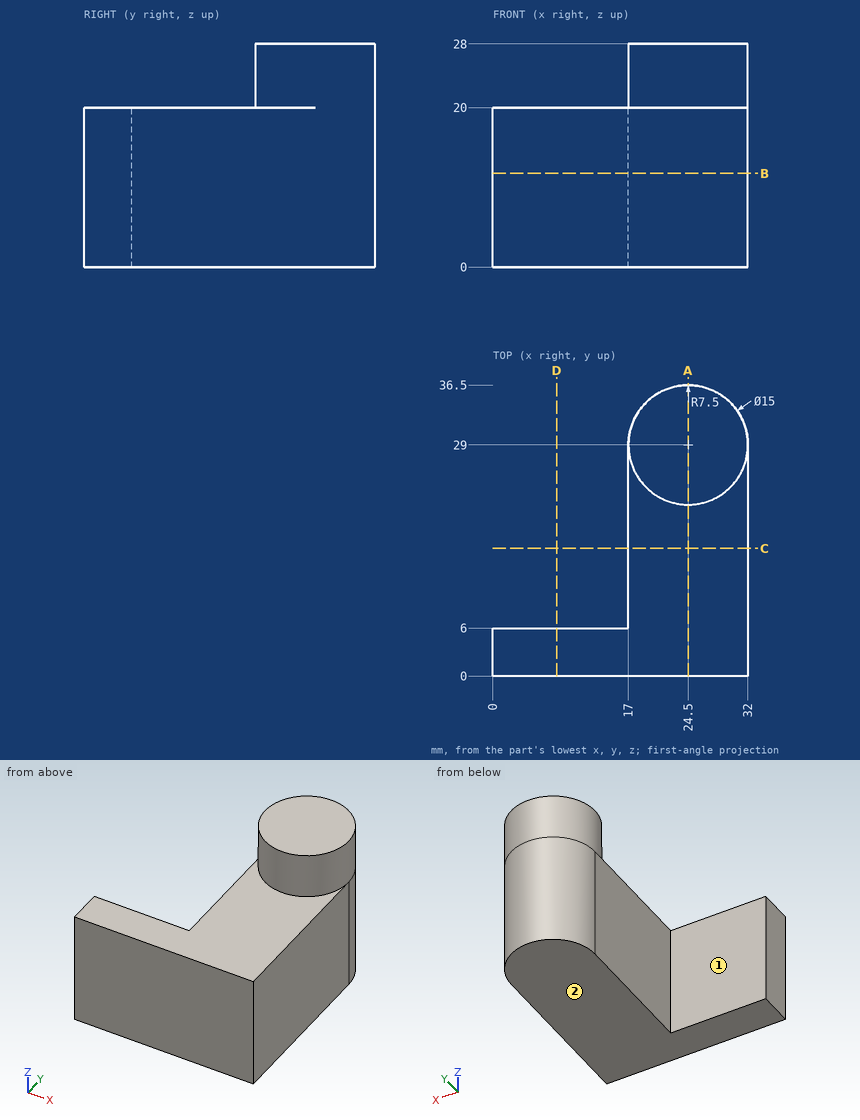
Study the drawing (mm; zero at the part's minimum x, y, z) and answer. A direction names the side the tool comes from. Give positions to 0.01 mm unless a question says otherwise; leave off trailing zeros. Order: outer loops, then holes, each group sorted by start corner. A loop starts at its lowest first (then second) coordinate and runs counter-clockwise, first axis right, second up. Notation, with made-up numbers: M 80,84 L 107,84 A17 cw 107,108 Z; hole C 61.25,83.5 d4. An arc over 180 degrees is marked long. Put each result on its own line as item: value. Start each with the question number.
Item 1: Flat-ended cylindrical pins translate along their axes: P1, Ø13.5, axis at x = 4.5, z = 7, coming from the +Y side; P2, Ø1.5, axis at y = 30, z = 9, coming from the +X side; P3, Ø10, axis at y = 14, z = 13.5, coming from the -X side. Find the tip coordinate at first contact, or state that the pin passes through.
Item 2: Which of the six approach directions +Z, -Z, +X, -X, +Y, -Y give full straight-line access (tool end or side, diameter ignored) to the marked faces 1 and 2?
Item 3: The part is cut by section B-B, the plane z = 11.75. Determine the outline of the cut face in (x, y).
Item 4: Find the intervals of material crossed by line 1 along Z through (x, y) = (7.5, 5); line 2 along Y through (x, z) = (16.5, 12); line 3 along X through (y, z) = (14, 12.25), in increasing order.
Item 5: The part is cut by section C-C, the plane y = 16. Determine the outline of the cut face in (x, z).
Item 6: The part is cut by section A-A, the plane x = 24.5. Determine the outline of the cut face in (y, z).
Item 7: The part is cut by section D-D, the plane x = 8. Determine the outline of the cut face in (y, z).
Answer key:
1. P1: stops at y = 6
1. P2: stops at x = 32
1. P3: stops at x = 17
2. face 1: +Z, -Z, -X, +Y
2. face 2: -Z, +X, -X, +Y, -Y
3. outline: M 0,0 L 32,0 L 32,29 A7.5 ccw 17,29 L 17,6 L 0,6 Z
4. line 1: z = 0 to 20
4. line 2: y = 0 to 6
4. line 3: x = 17 to 32
5. outline: M 17,0 L 32,0 L 32,20 L 17,20 Z
6. outline: M 0,0 L 36.5,0 L 36.5,28 L 21.5,28 L 21.5,20 L 0,20 Z
7. outline: M 0,0 L 6,0 L 6,20 L 0,20 Z
